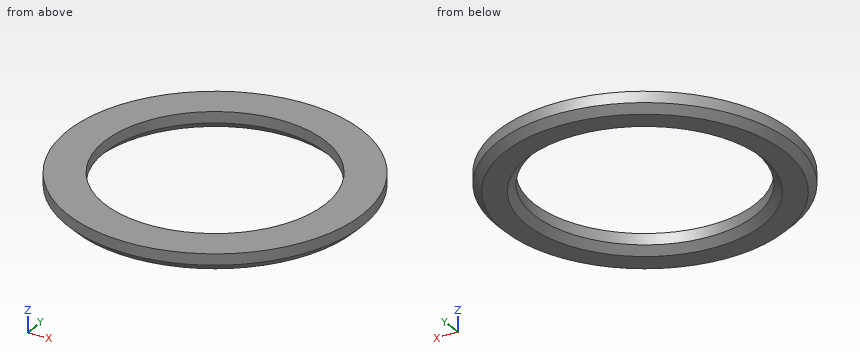
Autodesk Fusion 360 part; units mm, degrees
sketch "Sketch1" plane through (0, 0, 0) normal (0, 0, 1) x (1, 0, 0)
  circle A0 centre (0, 0) radius 20
  circle A1 centre (0, 0) radius 15
  dimension "d1" = 40
  dimension "d2" = 30
extrude "Extrude1" add sketch "Sketch1" along normal blind 2.5
chamfer "Chamfer1" distance 1 angle 45 1 edges at (-18.6465, -7.2323, 0)
chamfer "Chamfer2" distance 1 angle 45 1 edges at (-13.9849, 5.4242, 0)
Geometry: final body of the model. Coordinates: model frame, mm. Round coordinates to 2 decimals unless told otherwise and drop trailing zeros. Order: outer loops, then holes, each group sorted by start corner. A loop starts at its lowest first (then second) coordinate and runs counter-clockwise, first axis right, second up. Notation, with made-up numbers: (-31.5, 32.25) -> (-4.5, 32.25) arc R23 ccw to (-4.5, 53.25) -> close; hole circle Ø1 at (36.5, -31.75). An arc over 180 degrees is marked (long way). Put each result on its own line as item: value. Start each with the question number.
Q1. Section A-A on y = 0. Return the cut outline in (x, z).
Q2. Section C-C on z = 1.6. Return the cut outline in (x, y), and give its area (3 significant figures).
Q3. Line query: probe 1 along Y at (x, z) = (0, 1.9); probe 2 along X at (y, z) = (-5.5, 1.3); probe 3 along X at (y, z) = (-9.5, 0.9). Output: solid intervals per line, ascending.
Q4. First-contact query: pin 1 (10 mm diameter, centred on x = 0.5, y = -14, fed in from +Z). Flat tip, straight axial feed; report the tip coordinate or a pass-through.
Ans:
1. outline: (-20, 1) -> (-19, 0) -> (-16, 0) -> (-15, 1) -> (-15, 2.5) -> (-20, 2.5) -> close; (15, 1) -> (16, 0) -> (19, 0) -> (20, 1) -> (20, 2.5) -> (15, 2.5) -> close
2. outline: circle Ø40 at (0, 0); hole circle Ø30 at (0, 0)
2. area: 550 mm2
3. probe 1: y = -20 to -15, 15 to 20
3. probe 2: x = -19.23 to -13.96, 13.96 to 19.23
3. probe 3: x = -17.49 to -11.74, 11.74 to 17.49
4. pin 1: stops at z = 2.5
